For this review, take the finished solid that the model builds, in its own axes (mm). A direction names the side the tool comes from. Coordinates: 2 decimals unless noted, no trailing zeros. Loops run counter-clockwise (first coordinate to the right, second up) from the corner with the lowest first, then second, coordinate; pieces in that order, holes last. Notation, with made-up numbers: (69, 80) - (121, 80) arc R16 cw to (121, 97) - close; hole circle Ø9 at (53, 72). An arc over 180 degrees is marked (long way). One line per item, written item: value. Start each with the question number.
1. For faces 1 (the face through (23, 6, 0)), 2 (the face through (-13, 20, -86)), list the 3-axis set-ups (+Z, -Z, +X, -X, +Y, -Y) from which the entire face can be reached by the end or side of a thin tool; tool diameter is ignored.
2. Take a section at C-C, the plane y = 7.5. State the section outline as (x, z) points, and give its area (3 significant figures).
3. To check wall thickness, follow line 1 (X direction, y = 29.5, z = -27.5); line 2 (Z direction, x = 0, y = 14.5); line 3 (Z direction, x = -21.5, y = 33.5). State the ranges of each line that lie inside material, in increasing order. Write a range as from..to.
4. Insertion check: pin 1 (4 mm diameter, centred on x = -20.5, y = 16, fed in from +Z); pin 2 (2 mm diameter, centred on x = -2, y = 13, fed in from +Z); pin 3 (5 mm diameter, centred on x = -11, y = 28.5, fed in from -Z). Each pin has a flat end and moves straight along its axis. Give the tip position at first contact, or say it passes through.
5. Take a section at D-D, the plane x = 0. State the section outline as (y, z) points.
6. Take a section at A-A, the plane z = -51.5. State the section outline as (x, y) points.
7. The part is to be moulded in two halves that separate along X. For faces 3 (the face through (-33, 20, -86)), 4 (the face through (-23, 6, 0)), 5 (the face through (13, 20, -84)), say which applies: released by +X, released by -X, zero draft, split by the parting line, or undercut.
8. Take a section at B-B, the plane y = 30. State the section outline as (x, z) points, and give its area (3 significant figures).
```python
from build123d import *

# Parameters (mm, degrees)
SKETCH1_W     = 20
SKETCH1_H     = 40
CHAMFER1_SIZE = 28


with BuildPart() as part:
    # Sweep1: sweep along a path in Sketch2
    with BuildLine(Plane(origin=(0, 0, 0), x_dir=(1, 0, 0), z_dir=(0, 1, 0))) as sweep1_path:
        Line((-13, 0), (-13, 170))
        ThreePointArc((-13, 170), (0, 183), (13, 170))
        Line((13, 170), (13, 0))
    # Sketch1 → Sweep1 (sweep)
    with BuildSketch(Plane.XY):
        with Locations((-23, 20)):
            Rectangle(SKETCH1_W, SKETCH1_H)
    sweep(path=sweep1_path.line)

    # Chamfer1
    chamfer1_edges = [part.edges().sort_by_distance(p)[0] for p in [
        (-23, 40, 0),
        (23, 40, 0),
    ]]
    chamfer(chamfer1_edges, length=CHAMFER1_SIZE)


solid = part.part
```
Solutions:
1. face 1: +Z, +X, -X, +Y, -Y
1. face 2: +Z, +Y, -Y
2. outline: (-33, -170) arc R33 ccw to (33, -170) - (33, 0) - (13, 0) - (13, -170) arc R13 cw to (-13, -170) - (-13, 0) - (-33, 0) - close
2. area: 8,250 mm2
3. line 1: -33..-13, 13..33
3. line 2: -203..-183
3. line 3: -195.03..-21.5
4. pin 1: z = -2
4. pin 2: z = -182.65
4. pin 3: z = -201.89
5. outline: (0, -203) - (40, -203) - (40, -183) - (0, -183) - close
6. outline: (-33, 0) - (-13, 0) - (-13, 40) - (-33, 40) - close; (13, 0) - (33, 0) - (33, 40) - (13, 40) - close
7. face 3: released by -X
7. face 4: zero draft
7. face 5: undercut
8. outline: (-33, -170) arc R33 ccw to (33, -170) - (33, -18) - (13, -18) - (13, -170) arc R13 cw to (-13, -170) - (-13, -18) - (-33, -18) - close
8. area: 7,530 mm2
